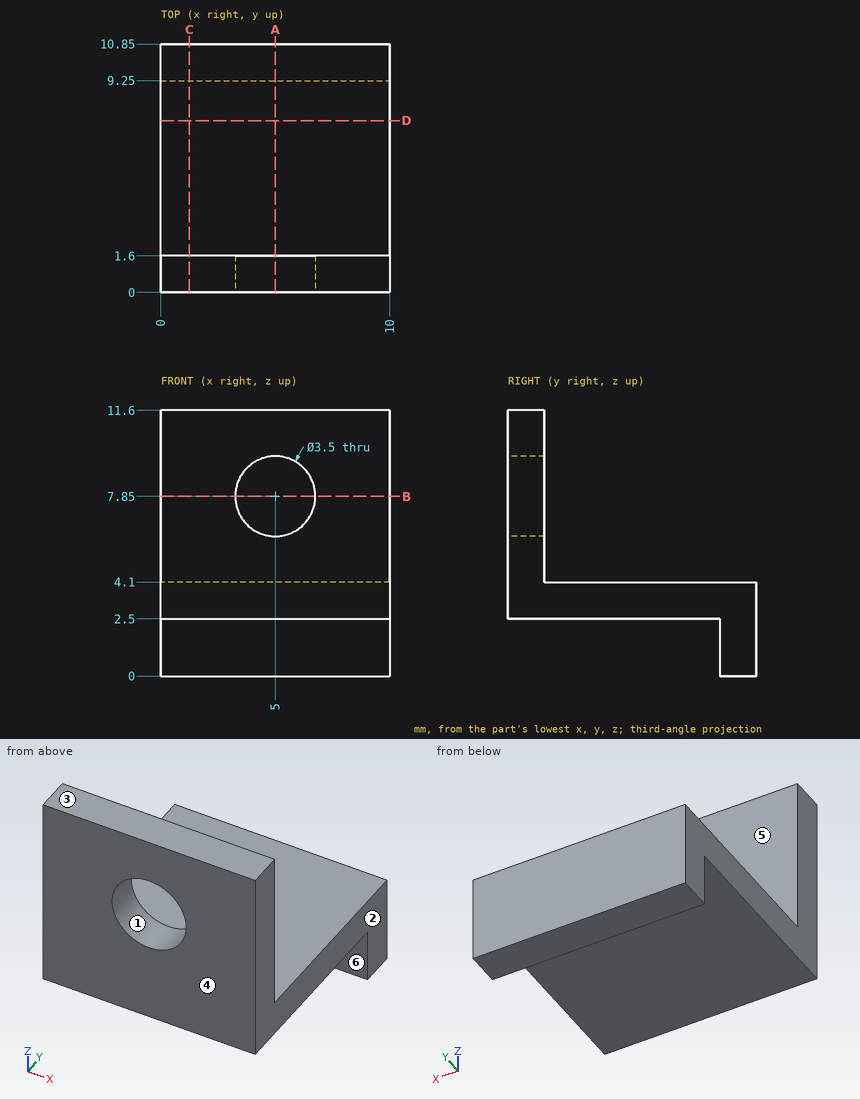
Can you work these out from the drawing? Everything is in mm from the part's minimum corner. A direction names the side the tool comes from. Give positions to 0.01 mm unless a question says otherwise; leave off trailing zeros. Write each loop counter-clockwise with the first axis right and the second up, starting at its lowest first coordinate (ties: lowest second). Pieces come first, ordered by that corner, then holes. Notation, with made-up numbers: M -19.75,10.25 L 17.25,10.25 A23 cw 17.25,44.25 Z; hole C 56.25,-38.5 d1. An arc over 180 degrees is marked long. Answer in a Markdown table with one row per item. Add a question column.
Item 1: Please list where these lines run through material, in increasing order: L1, parallel to Z at x = 5, y = 1.15; L2, parallel to X at y = 0.95, z = 7.85; L3, parallel to Z at x = 7.75, y = 8.5.
Item 2: Imagine slicing it at B-B, the plane z = 7.85. Write out the boundary of the cut face in (x, y), plus the area to 3 significant figures.
Item 3: On a 3-axis mill with a long thin cutter (end or side, diameter ignored), from which of +Z, -Z, +X, -X, +Y, -Y can I reach the whole of each face in a straight line? I mean the marked faces 4, 5 and 6. Say none if no direction works.
Item 4: Imagine slicing it at A-A, the plane x = 5. Write out the boundary of the cut face in (y, z).
Item 5: Imagine slicing it at C-C, the plane x = 1.25. Write out the boundary of the cut face in (y, z), plus the area to 3 significant figures.
Item 6: For pin 1 Ø6 at (x, y) = (1.5, 7.5) entering from +Z; pin 2 Ø3 at (x, y) = (2.5, 4) entering from -Z; pin 3 Ø2 at (x, z) = (3.5, 1) entering from -Y, each with a flat end and sliding along its axis, tell me the tip position at first contact or that it passes through.
Item 7: We'd pull the mould along X, two halves only. Please class the marked faces 1, 2 and 3: released by +X, released by -X, zero draft, split by the parting line, or undercut.
Item 8: Imagine slicing it at D-D, the plane y = 7.5. Write out the boundary of the cut face in (x, z).
Evaluation:
| question | item | result |
|---|---|---|
| 1 | L1 | z = 2.5 to 6.1, 9.6 to 11.6 |
| 1 | L2 | x = 0 to 3.25, 6.75 to 10 |
| 1 | L3 | z = 2.5 to 4.1 |
| 2 | outline | M 0,0 L 3.25,0 L 3.25,1.6 L 0,1.6 Z; M 6.75,0 L 10,0 L 10,1.6 L 6.75,1.6 Z |
| 2 | area | 10.4 mm² |
| 3 | face 4 | +Z, -Z, +X, -X, -Y |
| 3 | face 5 | +Z, +X, -X, +Y |
| 3 | face 6 | -Z, +X, -X, -Y |
| 4 | outline | M 0,2.5 L 9.25,2.5 L 9.25,0 L 10.85,0 L 10.85,4.1 L 1.6,4.1 L 1.6,6.1 L 0,6.1 Z; M 0,9.6 L 1.6,9.6 L 1.6,11.6 L 0,11.6 Z |
| 5 | outline | M 0,2.5 L 9.25,2.5 L 9.25,0 L 10.85,0 L 10.85,4.1 L 1.6,4.1 L 1.6,11.6 L 0,11.6 Z |
| 5 | area | 33.4 mm² |
| 6 | pin 1 | stops at z = 4.1 |
| 6 | pin 2 | stops at z = 2.5 |
| 6 | pin 3 | stops at y = 9.25 |
| 7 | face 1 | undercut |
| 7 | face 2 | released by +X |
| 7 | face 3 | zero draft |
| 8 | outline | M 0,2.5 L 10,2.5 L 10,4.1 L 0,4.1 Z |
